The drawing under review shows one solid part. Ordinate dimensions are in mm from its lowest x, y, z. A direction names the side the tool comes from. Give positions to 0.01 mm unless a question says otherwise; leave off trailing zeros. Order: outer loops, then holes, each group sorted by start corner. A loop starts at its lowest first (then second) coordinate and runs counter-clockwise, first axis right, second up. Notation, with made-up numbers: (-38, 55) -> (4, 55) arc R9 cw to (4, 70) -> close; hole circle Ø4 at (74.5, -22.75). An arc over 180 degrees is marked (long way). Return JSON: item names as keys, results as strings. Group by question number.
1) To check wall thickness, follow line 1 along X through (y, z) = (9.5, 19) (1 decimal); line 2 along Y through (x, z) = (9, 11) (1 decimal); line 3 along Y through (x, z) = (8.5, 9.5) (1 decimal). State the ranges of each line that lie inside material, in increasing order.
2) Add section D-D (z = 2). Give the boundary of the cut face in (x, y) (1 decimal), then the cut area to 3 significant figures.
3) Add section C-C (y = 9.75). Give the boundary of the cut face in (x, z) (1 decimal).
4) For the marked faces 1, 2 and 3, list the 3-axis set-ups (+Z, -Z, +X, -X, +Y, -Y) from which the entire face can be reached by the end or side of a thin tool; tool diameter is ignored.
5) Add section A-A (z = 16.5). Give the boundary of the cut face in (x, y) (1 decimal).
6) Insertion check: P1, Ø6.5, axis at x = 17.5, z = 10.5, coming from the +Y side; P2, Ø1, axis at x = 7.5, z = 12.5, coming from the -Y side; P3, Ø6, axis at x = 5.5, y = 13, coming from the -Z side. Each pin has a flat end and moves straight along its axis. Give the tip position at first contact, or say it passes through.
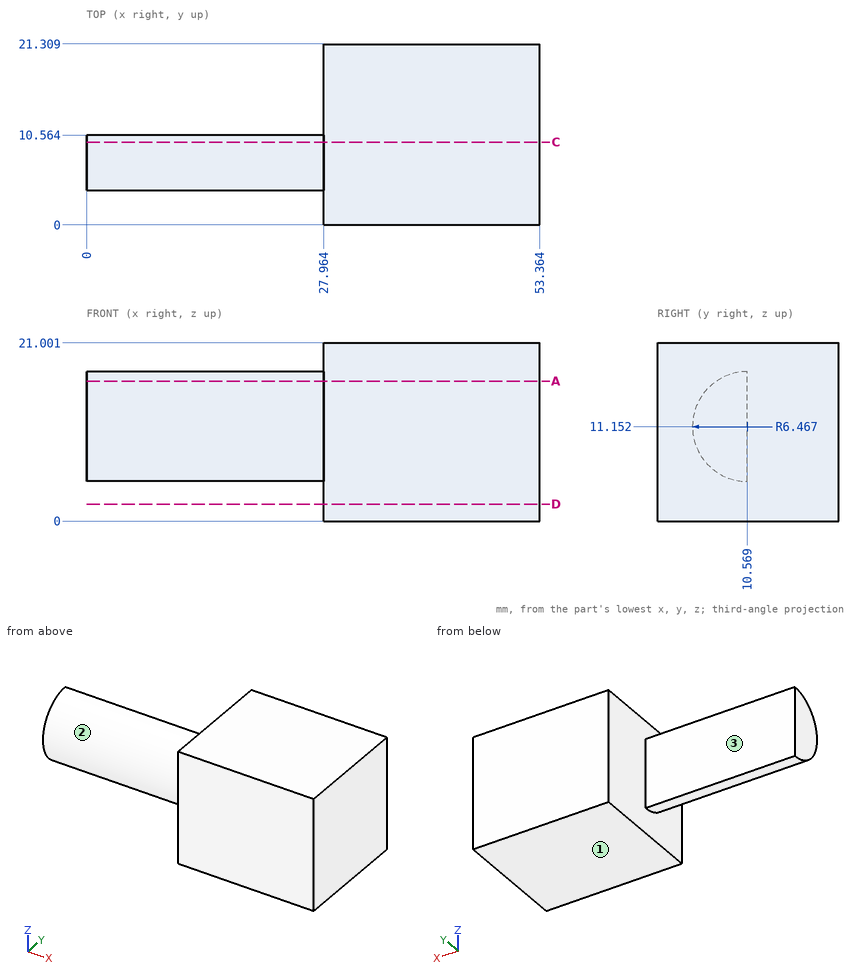
Evaluation:
{
 "1": {"line 1": "28 to 53.4", "line 2": "4.1 to 10.6", "line 3": "4.3 to 10.6"},
 "2": {"outline": "(28, 0) -> (53.4, 0) -> (53.4, 21.3) -> (28, 21.3) -> close", "area": "541 mm^2"},
 "3": {"outline": "(0, 4.7) -> (28, 4.7) -> (28, 0) -> (53.4, 0) -> (53.4, 21) -> (28, 21) -> (28, 17.6) -> (0, 17.6) -> close"},
 "4": {"face 1": "-Z, +X, -X, +Y, -Y", "face 2": "-X, -Y", "face 3": "+Z, -Z, -X, +Y"},
 "5": {"outline": "(0, 6.9) -> (28, 6.9) -> (28, 0) -> (53.4, 0) -> (53.4, 21.3) -> (28, 21.3) -> (28, 10.6) -> (0, 10.6) -> close"},
 "6": {"P1": "y = 10.56", "P2": "y = 4.16", "P3": "z = 4.69"}
}
